```python
from build123d import *

# Parameters (mm, degrees)
SKETCH1_R           = 5
BASEHEAD_DEPTH      = 6
SKETCH2_R           = 3
BASEBODY_DEPTH      = 10
HEXAGONSOCKET_DEPTH = 3
TOPFILLET_R         = 0.75
CHAMFER1_SIZE       = 0.25
LPATTERN10_COUNT    = 15
LPATTERN10_PITCH    = 0.6498
SKETCH_1_W          = 12.577775012
SKETCH_1_H          = 7.589665947
CUT_EXTRUDE_1_DEPTH = 2


with BuildPart() as part:
    # Sketch1 → BaseHead (new body)
    with BuildSketch(Plane(origin=(0, 0, 0), x_dir=(0, 0, -1), z_dir=(1, 0, 0))):
        Circle(SKETCH1_R)
    extrude(amount=BASEHEAD_DEPTH)

    # Sketch2 → BaseBody (add)
    with BuildSketch(Plane(origin=(6, 0, 0), x_dir=(0, 0, -1), z_dir=(1, 0, 0))):
        Circle(SKETCH2_R)
    extrude(amount=BASEBODY_DEPTH)

    # Sketch3 → HexagonSocket (cut)
    with BuildSketch(Plane(origin=(0, 0, 0), x_dir=(0, 0, -1), z_dir=(1, 0, 0))):
        Polygon((2.886751346, 0), (1.443375673, 2.5), (-1.443375673, 2.5), (-2.886751346, 0), (-1.443375673, -2.5), (1.443375673, -2.5), align=None)
    extrude(amount=HEXAGONSOCKET_DEPTH, mode=Mode.SUBTRACT)

    # Sketch4 → Cut-Revolve1 (revolve, cut)
    with BuildSketch(Plane(origin=(-4.19613823, 0.75, 0), x_dir=(-1, 0, 0), z_dir=(0, 0, 1))):
        Polygon((-7.19613823, 3.25), (-8.639513903, 0.75), (-7.19613823, 0.75), align=None)
    revolve(axis=Axis((0.838992387, 0, 0), (-1, 0, 0)), mode=Mode.SUBTRACT)

    # TopFillet
    topfillet_edges = [part.edges().sort_by_distance(p)[0] for p in [
        (0, 0, 5),
    ]]
    fillet(topfillet_edges, radius=TOPFILLET_R)

    # Chamfer1
    chamfer1_edges = [part.edges().sort_by_distance(p)[0] for p in [
        (16, 0, 3),
    ]]
    chamfer(chamfer1_edges, length=CHAMFER1_SIZE)

    # Sketch5 → Cut-Revolve10 (revolve, cut)
    with BuildSketch(Plane.XY):
        Polygon((15.75, 2.531047244), (16.02075, 3), (16.02075, 3.5415), (15.47925, 3.5415), (15.47925, 3), align=None)
    cut_revolve10 = revolve(axis=Axis((0, 0, 0), (1, 0, 0)), mode=Mode.SUBTRACT)

    # LPattern10: Cut-Revolve10 ×15
    with Locations(*[(-i * LPATTERN10_PITCH, 0, 0) for i in range(1, LPATTERN10_COUNT)]):
        add(cut_revolve10, mode=Mode.SUBTRACT)

    # 草图1 → 切除-拉伸1 (cut)
    with BuildSketch(Plane(origin=(16, 0, 0), x_dir=(0, 0, -1), z_dir=(1, 0, 0))):
        with Locations((-0.655764338, 0.333257287)):
            Rectangle(SKETCH_1_W, SKETCH_1_H)
    extrude(amount=-CUT_EXTRUDE_1_DEPTH, mode=Mode.SUBTRACT)

    # 草图2 → 切除-旋转1 (revolve, cut)
    with BuildSketch(Plane.XY):
        Polygon((14, 2.510742744), (13.709985541, 3.124600146), (14, 3.124600146), align=None)
    revolve(axis=Axis((0, 0, 0), (1, 0, 0)), mode=Mode.SUBTRACT)


solid = part.part
```
For this review, take the finished solid that the model builds, in its own axes (mm). A direction names the side the tool comes from. Coordinates: 2 decimals unless noted, no trailing zeros. Return JSON: item names as keys, results as strings. Group by question number.
(1) To check wall thickness, follow L1, parallel to Y at x = 1.75, z = 0.5; L2, parallel to Z at x = 2.5, y = -1.75; L3, parallel to Y at x = 10.5, z = 0.25. State the ranges of each line that lie inside material, in increasing order.
(2) Tool access review of faces 1 (the flat face through (1.479, -1.233, 2.175)), 2 (the cylindrical face through (6.19, -1.15, -2.77)): name each direction out of +Z, -Z, +X, -X, +Y, -Y from which nothing blocks a thin tool from reaching the whole face with its end or side.
(3) For pin 1 Ø1 at (x, z) = (8.5, -4) entering from +Y; pin 2 Ø0.6 at (y, z) = (0.5, 2.5) entering from -X; pin 3 Ø4 at (x, z) = (3.5, -3) entering from -Y; pin 4 Ø5 at (x, y) = (1.5, 3) entering from -Z, all flat-tipped, find the tip position at first contact; note any pin that passes through.
Results below:
{
 "1": {"L1": "y = -4.97 to -2.5, 2.5 to 4.97", "L2": "z = -4.68 to -1.88, 1.88 to 4.68", "L3": "y = -2.61 to 2.61"},
 "2": {"face 1": "-X", "face 2": "+X"},
 "3": {"pin 1": "passes through", "pin 2": "stops at x = 0", "pin 3": "stops at y = -4.9", "pin 4": "stops at z = -4.97"}
}
